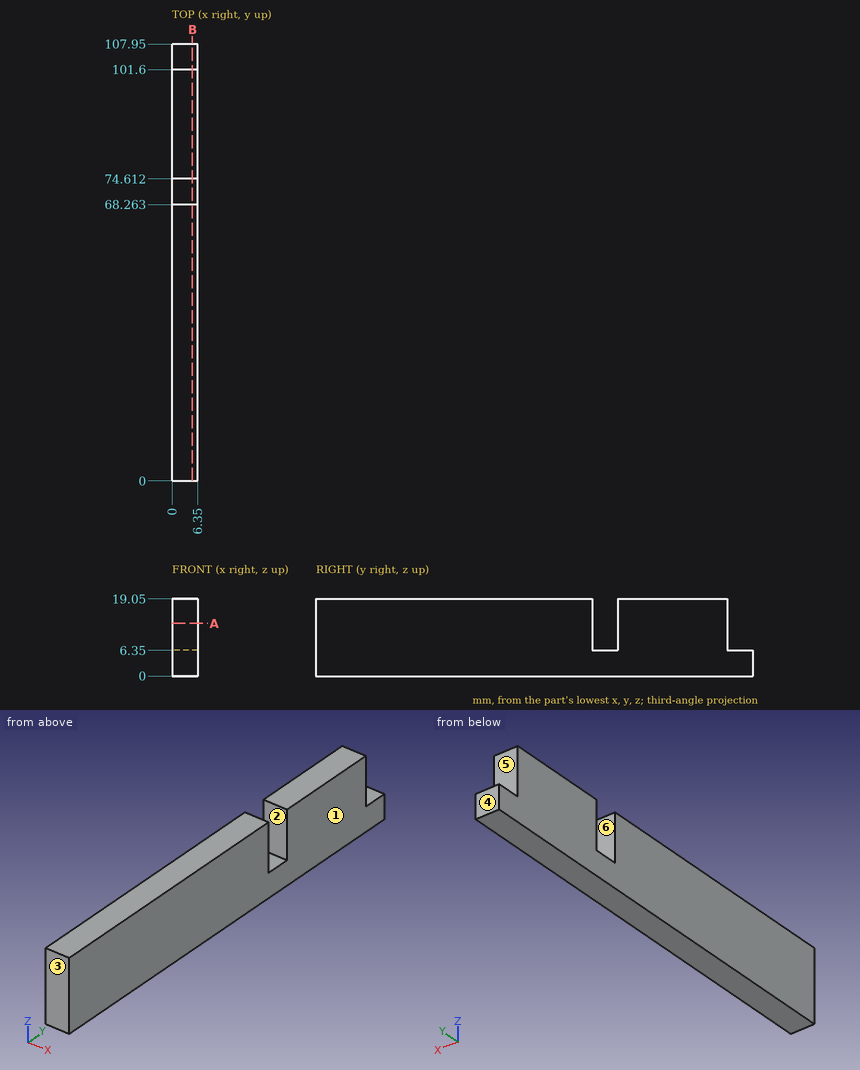
Check sheet for the drawn part. Datum: minimum x, y, z corner. Units: mm. A direction names the side the tool comes from. Round coordinates to 2 decimals unless told otherwise and drop trailing zeros. Write each loop counter-clockwise with the first axis right and the second up, starting at its lowest first coordinate (ties: lowest second). Pieces come first, ordered by that corner, then holes. Notation, with made-up numbers: (-6.5, -21.5) - (19.5, -21.5) arc R24 ccw to (19.5, 9.5) - close; hole circle Ø6 at (43, 24.5). An arc over 180 degrees is marked (long way). Return JSON: item names as keys, results as strings.
Q1. Scan lines: L1, parallel to Y at x = 4.75, z = 8.75; L2, parallel to Z at x = 5.5, y = 102. Record each from-to range of solid material in increasing order. Write a range as from..to.
Returned:
{"L1": "y = 0..68.26, 74.61..101.6", "L2": "z = 0..6.35"}
Q2. Depth check by flat-ended pin: P1, Ø1.9, axis at x = 2, y = 72.5, coming from the +Z side; P2, Ø2, axis at x = 5, z = 10.5, coming from the -Y side. Enter the tip coordinate at first touch or a pass-through.
Returned:
{"P1": "stops at z = 6.35", "P2": "stops at y = 0"}
Q3. Cross-section at B-B (x = 5). Record the boundary of the cut face in (y, z).
Returned:
{"outline": "(0, 0) - (107.95, 0) - (107.95, 6.35) - (101.6, 6.35) - (101.6, 19.05) - (74.61, 19.05) - (74.61, 6.35) - (68.26, 6.35) - (68.26, 19.05) - (0, 19.05) - close"}
Q4. Access from +Z, -Z, +X, -X, +Y, -Y to the whole of each face (thin tool, end or side, straight path). Record for the marked faces 4, 5 and 6.
Returned:
{"face 4": "+Z, -Z, +X, -X, +Y", "face 5": "+Z, +X, -X, +Y", "face 6": "+Z, +X, -X"}
Q5. Cross-section at A-A (z = 13). Record the boundary of the cut face in (x, y).
Returned:
{"outline": "(0, 0) - (6.35, 0) - (6.35, 68.26) - (0, 68.26) - close; (0, 74.61) - (6.35, 74.61) - (6.35, 101.6) - (0, 101.6) - close"}
Q6. Draft check along Y on the marked faces 1, 2 and 3. Enter one of: released by +Y, released by -Y, zero draft, split by the parting line, or undercut.
Returned:
{"face 1": "zero draft", "face 2": "undercut", "face 3": "released by -Y"}
